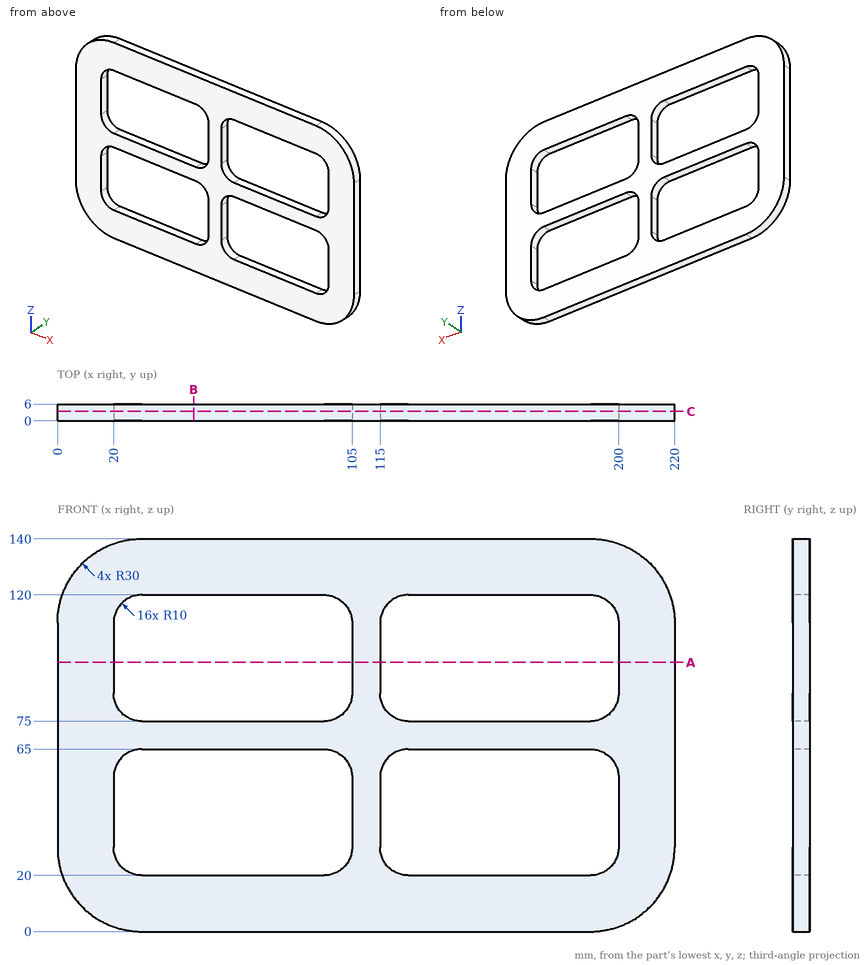
Job drawing, mm, ordinate dimensions from the low corner. One solid piece. Round coordinates to 2 decimals unless told otherwise and drop trailing zeros. Order: outer loops, then holes, each group sorted by start corner. A loop starts at its lowest first (then second) coordinate and runs counter-clockwise, first axis right, second up. Notation, with made-up numbers: M 10.25,-20.5 L 48.25,-20.5 A23 cw 48.25,12.5 Z; hole C -4,-33.5 d3. An arc over 180 degrees is marked long. Write each question's results on one line, items separated by ' | '. Start each with the question number.
(1) Saw through at A-A, the plane z = 96. Give the cut face in (x, y), then the cut area to 3 significant figures.
(2) Saw through at C-C, the plane y = 3.4. State how many separate pieces and enclosed holes the cut face has, then the cut area to 3 significant figures.
(3) Saw through at B-B, the plane x = 48.5. Give the cut face in (y, z).
(4) Probe probe 1 along X at (y, z) = (1.5, 37.5); probe 2 along Z at (x, y) = (141.5, 4.5); probe 3 along X at (y, z) = (1.4, 76). List the from-to ranges inside material, lowest first. Write a range as from..to.
Established:
1) outline: M 0,0 L 20,0 L 20,6 L 0,6 Z; M 105,0 L 115,0 L 115,6 L 105,6 Z; M 200,0 L 220,0 L 220,6 L 200,6 Z | area: 300 mm^2
2) separate pieces: 1 | enclosed holes: 4 | area: 15,100 mm^2
3) outline: M 0,0 L 6,0 L 6,20 L 0,20 Z; M 0,65 L 6,65 L 6,75 L 0,75 Z; M 0,120 L 6,120 L 6,140 L 0,140 Z
4) probe 1: x = 0..20, 105..115, 200..220 | probe 2: z = 0..20, 65..75, 120..140 | probe 3: x = 0..25.64, 99.36..120.64, 194.36..220
